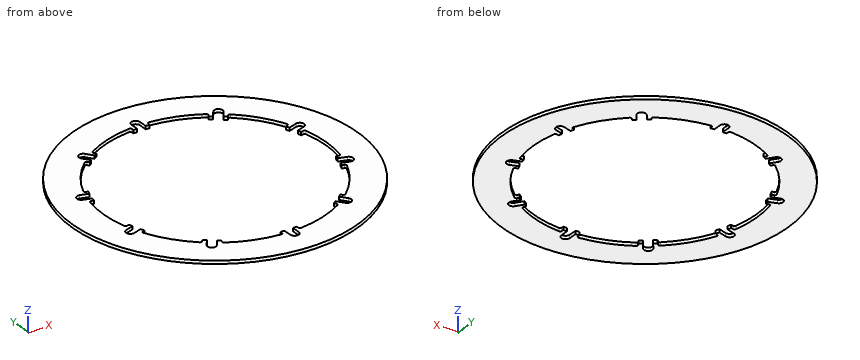
```python
from build123d import *

# Parameters (mm, degrees)
SKETCH1_R           = 212.725
BOSS_EXTRUDE1_DEPTH = 4.7625
SKETCH8_R           = 166.37
CUT_EXTRUDE1_DEPTH  = 4.7625
CUT_EXTRUDE3_DEPTH  = 4.7625
CIRPATTERN1_COUNT   = 10
BOSS_EXTRUDE2_START = -4.7625
BOSS_EXTRUDE2_DEPTH = 4.7625
CIRPATTERN2_COUNT   = 10


with BuildPart() as part:
    # Sketch1 → Boss-Extrude1 (new body)
    with BuildSketch(Plane.XY):
        with Locations(Location((0, 0, 0), (0, 0, 180))):
            Circle(SKETCH1_R)
    extrude(amount=BOSS_EXTRUDE1_DEPTH)

    # Sketch8 → Cut-Extrude1 (cut)
    with BuildSketch(Plane(origin=(0, 0, 0), x_dir=(-1, 0, 0), z_dir=(0, 0, -1))):
        Circle(SKETCH8_R)
    extrude(amount=-CUT_EXTRUDE1_DEPTH, mode=Mode.SUBTRACT)

    # Sketch9 → Cut-Extrude3 (cut)
    with BuildSketch(Plane(origin=(0, 0, 0), x_dir=(-1, 0, 0), z_dir=(0, 0, -1))):
        with BuildLine():
            ThreePointArc((6.35, 172.72), (0, 179.07), (-6.35, 172.72))
            Line((-6.35, 172.72), (6.35, 172.72))
        make_face()
        with BuildLine():
            Line((6.35, 172.72), (-6.35, 172.72))
            ThreePointArc((-6.35, 172.72), (-4.490128088, 168.229871967), (-7.7e-08, 166.37))
            ThreePointArc((-7.7e-08, 166.37), (4.490128033, 168.229871912), (6.35, 172.72))
        make_face()
        with BuildLine():
            ThreePointArc((-7.7e-08, 166.37), (3.175578494, 166.339690397), (6.35, 166.248772627))
            Line((6.35, 166.248772627), (6.35, 172.72))
            ThreePointArc((6.35, 172.72), (4.490128033, 168.229871912), (-7.7e-08, 166.37))
        make_face()
        with BuildLine():
            Line((-6.35, 172.72), (-6.35, 166.248772627))
            ThreePointArc((-6.35, 166.248772627), (-3.175578572, 166.339690395), (-7.7e-08, 166.37))
            ThreePointArc((-7.7e-08, 166.37), (-4.490128088, 168.229871967), (-6.35, 172.72))
        make_face()
    cut_extrude3 = extrude(amount=-CUT_EXTRUDE3_DEPTH, mode=Mode.SUBTRACT)

    # CirPattern1: Cut-Extrude3 ×10 about axis
    cirpattern1_axis = Axis((0, 0, 0), (0, 0, 1))
    for i in range(1, CIRPATTERN1_COUNT):
        add(cut_extrude3.rotate(cirpattern1_axis, i * 360 / CIRPATTERN1_COUNT), mode=Mode.SUBTRACT)

    # Sketch11 → Boss-Extrude2 (add)
    with BuildSketch(Plane.XY.offset(4.7625).offset(BOSS_EXTRUDE2_START)):
        with BuildLine():
            Line((-12.157574607, 163.359431727), (-11.893810893, 159.832075437))
            ThreePointArc((-11.893810893, 159.832075437), (-9.123274415, 160.014127314), (-6.35, 160.148158204))
            Line((-6.35, 160.148158204), (-6.35, 166.248772627))
            ThreePointArc((-6.35, 166.248772627), (-10.637673325, 166.029566061), (-14.918262729, 165.699795827))
            ThreePointArc((-14.918262729, 165.699795827), (-13.048012002, 165.107506557), (-12.157574607, 163.359431727))
        make_face()
        with BuildLine():
            ThreePointArc((14.986366689, 165.693650191), (10.671793481, 166.027376429), (6.35, 166.248772627))
            Line((6.35, 166.248772627), (6.35, 160.148158204))
            ThreePointArc((6.35, 160.148158204), (9.156780546, 160.012213428), (11.960746269, 159.827080386))
            Line((11.960746269, 159.827080386), (12.224649917, 163.353528381))
            ThreePointArc((12.224649917, 163.353528381), (13.1155312, 165.101840374), (14.986366689, 165.693650191))
        make_face()
    boss_extrude2 = extrude(amount=BOSS_EXTRUDE2_DEPTH)

    # CirPattern2: Boss-Extrude2 ×10 about axis
    cirpattern2_axis = Axis((0, 0, 0), (0, 0, 1))
    for i in range(1, CIRPATTERN2_COUNT):
        add(boss_extrude2.rotate(cirpattern2_axis, i * 360 / CIRPATTERN2_COUNT))


solid = part.part
```
Input: part model. Units: mm. Frame: model coordinates. Give positions to 0.01 mm unless a question says otherwise; leave off trailing zeros. Order: outer loops, then holes, each group sorted by start corner. A loop starts at its lowest first (then second) coordinate and runs counter-clockwise, first axis right, second up. Notation, with made-up numbers: M 50.5,75 L 74.5,75 A20 ccw 74.5,79 Z; hole C 20.5,41 d7. An arc over 180 degrees is marked long. One line per question, with ' | ' between items. Start each with the question number.
1. Section query A-A (x = 0). Return the cut outline in (y, z) (1 decimal).
2. Section query B-B (y = -80.5). Return the cut outline in (x, z), and give its area (3 significant figures).
3. Material intervals for probe 1 along Y at (x, z) = (85.5, 0.3); probe 2 along Y at (x, z) = (92.5, 3.6); probe 3 along X at (y, z) = (36, 3.45), sorted ascending. Write a range as [from, to].
4. First-contact query: pin 1 Ø1.4 at (y, z) = (168.5, 2) entering from -X; pin 2 Ø3 at (x, y) = (-155, 46) entering from +Z; pin 3 Ø1.4 at (y, z) = (-164.5, 2.5) entering from -X. Flat tips, straight axial feed; report the tip coordinate or a pass-through.
Here are the results:
1) outline: M -212.7,0 L -179.1,0 L -179.1,4.8 L -212.7,4.8 Z; M 179.1,0 L 212.7,0 L 212.7,4.8 L 179.1,4.8 Z
2) outline: M -196.91,0 L -145.6,0 L -145.6,4.76 L -196.91,4.76 Z; M 145.6,0 L 196.91,0 L 196.91,4.76 L 145.6,4.76 Z | area: 489 mm²
3) probe 1: [-194.79, -142.7], [-138.33, -135.56], [135.56, 138.2], [142.71, 194.79] | probe 2: [-191.56, -138.12], [138.12, 191.56] | probe 3: [-209.66, -162.43], [162.43, 209.66]
4) pin 1: x = -130.75 | pin 2: through | pin 3: x = -135.73
